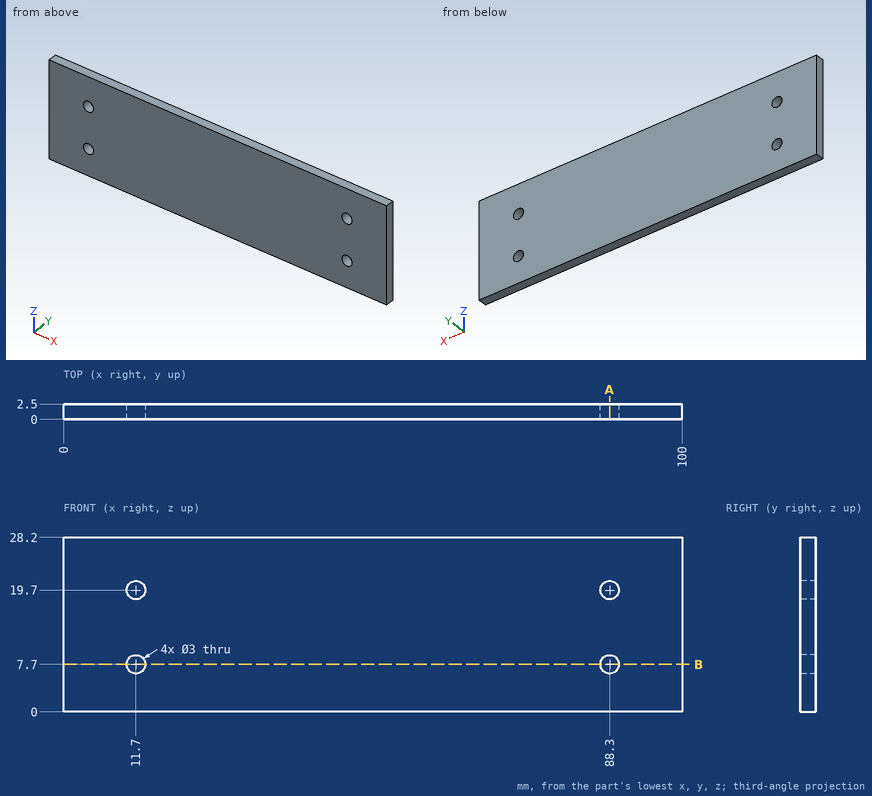
Job drawing, mm, ordinate dimensions from the low corner. One solid piece. Round coordinates to 2 decimals unless told otherwise and drop trailing zeros. Write each loop counter-clockwise with the first axis right and the second up, starting at its lowest first coordinate (ties: lowest second). Pieces come first, ordered by that corner, then holes.
1) Band-saw the part on A-A, the plane x = 88.3. List the corners of the cut face in (y, z), and give its area (3 significant figures).
2) Drill centre lines: probe 1 along Z at (x, y) = (88.3, 1); probe 2 along Z at (x, y) = (10.5, 2.25); probe 3 along X at (y, z) = (1.4, 20.5). Where is each one in solid material? Low to high.
3) Band-saw the part on B-B, the plane z = 7.7. List the corners of the cut face in (x, y).
4) Pin check, flat tip, straight feed: pin 1 (1.8 mm diameter, centred on x = 88.3, z = 7.7, fed in from +Y). Stop position of the tip, or through.
Ans:
1. outline: (0, 0) - (2.5, 0) - (2.5, 6.2) - (0, 6.2) - close; (0, 9.2) - (2.5, 9.2) - (2.5, 18.2) - (0, 18.2) - close; (0, 21.2) - (2.5, 21.2) - (2.5, 28.2) - (0, 28.2) - close
1. area: 55.5 mm2
2. probe 1: z = 0 to 6.2, 9.2 to 18.2, 21.2 to 28.2
2. probe 2: z = 0 to 6.8, 8.6 to 18.8, 20.6 to 28.2
2. probe 3: x = 0 to 10.43, 12.97 to 87.03, 89.57 to 100
3. outline: (0, 0) - (10.2, 0) - (10.2, 2.5) - (0, 2.5) - close; (13.2, 0) - (86.8, 0) - (86.8, 2.5) - (13.2, 2.5) - close; (89.8, 0) - (100, 0) - (100, 2.5) - (89.8, 2.5) - close
4. pin 1: passes through
